For this review, take the finished solid that the model builds, in its own axes (mm). Face numbers are marked on the shaded views. Coordinates: 2 decimals unless noted, no trailing zeros. Loops run counter-clockwise (first coordinate to the right, second up) from the corner with the lowest first, then second, coordinate; pieces in that order, holes last. Notation, with made-up numbers: M 75.5,31.25 L 82.5,31.25 A26 cw 82.5,67.25 Z; hole C 72,34 d10. An arc over 180 degrees is marked long. Use one line per item in the form item = value.
```python
from build123d import *

# Parameters (mm, degrees)
BOSS_EXTRUDE1_DEPTH        = 12.7
SKETCH2_R                  = 25.4
CUT_EXTRUDE1_DEPTH         = 82.814026915
F_7_0_201_DIAMETER_HOLE1_D = 5.1054
CIRPATTERN1_COUNT          = 4


with BuildPart() as part:
    # Sketch1 → Boss-Extrude1 (new body)
    with BuildSketch(Plane(origin=(0, 0, 0), x_dir=(1, 0, 0), z_dir=(0, 1, 0))):
        Polygon((0, -57.15), (57.15, 0), (0, 57.15), (-57.15, 0), align=None)
    extrude(amount=BOSS_EXTRUDE1_DEPTH)

    # Sketch2 → Cut-Extrude1 (cut, through all)
    with BuildSketch(Plane(origin=(0, 12.7, 0), x_dir=(1, 0, 0), z_dir=(0, 1, 0))):
        with Locations(Location((0, 0, 0), (0, 0, 270))):
            Circle(SKETCH2_R)
    extrude(amount=-CUT_EXTRUDE1_DEPTH, mode=Mode.SUBTRACT)

    # #7 (0.201) Diameter Hole1 (through all)
    with Locations(Plane(origin=(0, 12.7, 0), x_dir=(-1, 0, 0), z_dir=(0, 1, 0))):
        with Locations((0, -50.8)):
            f_7_0_201_diameter_hole1 = Hole(F_7_0_201_DIAMETER_HOLE1_D / 2)

    # CirPattern1: #7 (0.201) Diameter Hole1 ×4 about axis
    cirpattern1_axis = Axis((0, 0, 0), (0, 1, 0))
    for i in range(1, CIRPATTERN1_COUNT):
        add(f_7_0_201_diameter_hole1.rotate(cirpattern1_axis, i * 360 / CIRPATTERN1_COUNT), mode=Mode.SUBTRACT)


solid = part.part
```
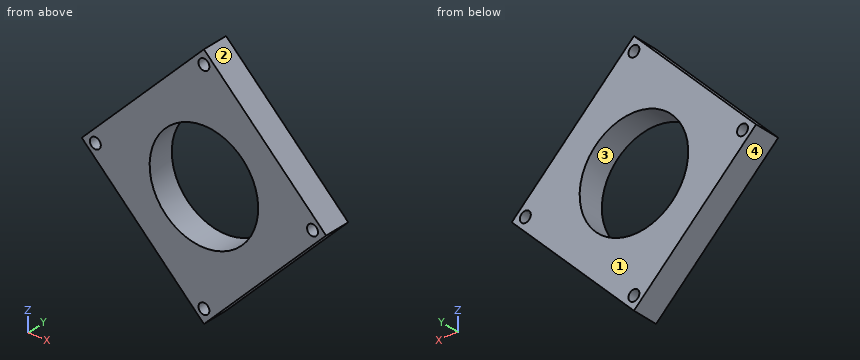
1. Consider section C-C on y = 3.25. Write out the cut boundary in (x, z), plus the area to 3 significant figures.
Computed values:
outline = M -57.15,0 L 0,-57.15 L 57.15,0 L 0,57.15 Z; hole C -50.8,0 d5.11; hole C 0,0 d50.8; hole C 0,-50.8 d5.11; hole C 0,50.8 d5.11; hole C 50.8,0 d5.11
area = 4,420 mm2
2. Wall thickness on line 1 along X through (y, z) = (9, 0); line 2 along X through (y, z) = (4.5, 50.8); line 3 along X through (y, z) = (10.5, -17): over which ranges is each line inside the solid? List them lowest first. Write a range as from..to.
Computed values:
line_1 = -57.15..-53.35, -48.25..-25.4, 25.4..48.25, 53.35..57.15
line_2 = -6.35..-2.55, 2.55..6.35
line_3 = -40.15..-18.87, 18.87..40.15
3. For pin 1 Ø1.5 at (y, z) = (9, 25) entering from -X; pin 2 Ø6 at (y, z) = (2, 23) entering from +X; pin 3 Ø2 at (y, z) = (3.5, 6) entering from +X, all flat-tipped, find the tip position at first contact; note any pin that passes through.
Computed values:
pin_1 = -32.9
pin_2 = 37.15
pin_3 = 52.15
4. Consider section A-A on z = -50.8. Write out the cut boundary in (x, y).
Computed values:
outline = M -6.35,0 L -2.55,0 L -2.55,12.7 L -6.35,12.7 Z; M 2.55,0 L 6.35,0 L 6.35,12.7 L 2.55,12.7 Z
5. Consider section B-B on x = -50.8. Write out the cut boundary in (y, z), plus the area to 3 significant figures.
Computed values:
outline = M 0,-6.35 L 12.7,-6.35 L 12.7,-2.55 L 0,-2.55 Z; M 0,2.55 L 12.7,2.55 L 12.7,6.35 L 0,6.35 Z
area = 96.5 mm2
6. Consider section D-D on x = 27.5. Write out the cut boundary in (y, z).
Computed values:
outline = M 0,-29.65 L 12.7,-29.65 L 12.7,29.65 L 0,29.65 Z
7. Draft analysis for pull direction Z (two halves, no side actions). For the marked faces 1, 2, 3 and 4, state which applies: +Z half, -Z half, draft (parallel to the pull), parting line (faces both ways), or undercut.
Computed values:
face_1 = draft
face_2 = +Z half
face_3 = undercut
face_4 = -Z half
